Read the model definition and answer for the solid it produces. Units are mm, in the model's axes. A direction names the side the tool comes from. Coordinates: 2 decimals unless noted, no trailing zeros. Loops run counter-clockwise (first coordinate to the right, second up) from the corner with the lowest first, then second, coordinate; pieces in that order, holes last. Notation, with made-up numbers: (-28.5, 27) -> (18.5, 27) arc R29 cw to (18.5, 59) -> close; hole circle Ø10 at (16, -32). An arc over 180 degrees is marked (long way). Answer in a Markdown table with one row per item.
```python
from build123d import *
from build123d.topology import SkipClean

# Parameters (mm, degrees)
BOSS_EXTRUDE1_START   = 100
SKETCH2_R             = 5
BOSS_EXTRUDE1_DEPTH   = 130
SKETCH2_R_2           = 50
SKETCH2_R_3           = 45
BOSS_EXTRUDE1_2_DEPTH = 130
SKETCH3_R             = 100
SKETCH3_R_2           = 50
CUT_EXTRUDE1_DEPTH    = 60
BOSS_EXTRUDE3_START   = 60
SKETCH4_R             = 5
BOSS_EXTRUDE3_DEPTH   = 60


with BuildPart() as part:
    # Sketch2 → Boss-Extrude1 (new body)
    with BuildSketch(Plane(origin=(0, 0, 0), x_dir=(0, 0, -1), z_dir=(0.5372996083468277, 0.8433914458128833, 0)).offset(BOSS_EXTRUDE1_START)):
        with BuildLine():
            ThreePointArc((198.707774346, 59.213708116), (179.337427943, 57.550334456), (177.879118885, 38.163471214))
            ThreePointArc((177.879118885, 38.163471214), (179.755724079, 33.196743881), (178.825393945, 27.96945842))
            ThreePointArc((178.825393945, 27.96945842), (172.5, 0), (178.825393945, -27.96945842))
            ThreePointArc((178.825393945, -27.96945842), (179.755724079, -33.196743881), (177.879118885, -38.163471214))
            ThreePointArc((177.879118885, -38.163471214), (179.337427943, -57.550334456), (198.707774346, -59.213708116))
            ThreePointArc((198.707774346, -59.213708116), (203.694081302, -57.389764479), (208.911229611, -58.375356167))
            ThreePointArc((208.911229611, -58.375356167), (237.5, -65), (266.088770389, -58.375356167))
            ThreePointArc((266.088770389, -58.375356167), (271.305918698, -57.389764479), (276.292225654, -59.213708116))
            ThreePointArc((276.292225654, -59.213708116), (295.662572057, -57.550334456), (297.120881115, -38.163471214))
            ThreePointArc((297.120881115, -38.163471214), (295.244275921, -33.196743881), (296.174606055, -27.96945842))
            ThreePointArc((296.174606055, -27.96945842), (302.5, 0), (296.174606055, 27.96945842))
            ThreePointArc((296.174606055, 27.96945842), (295.244275921, 33.196743881), (297.120881115, 38.163471214))
            ThreePointArc((297.120881115, 38.163471214), (295.662572057, 57.550334456), (276.292225654, 59.213708116))
            ThreePointArc((276.292225654, 59.213708116), (271.305918698, 57.389764479), (266.088770389, 58.375356167))
            ThreePointArc((266.088770389, 58.375356167), (237.5, 65), (208.911229611, 58.375356167))
            ThreePointArc((208.911229611, 58.375356167), (203.694081302, 57.389764479), (198.707774346, 59.213708116))
        make_face()
        with Locations(Location((190, -47, 0), (0, 0, 90))):
            Circle(SKETCH2_R, mode=Mode.SUBTRACT)
        with Locations(Location((285, -47, 0), (0, 0, 90))):
            Circle(SKETCH2_R, mode=Mode.SUBTRACT)
        with Locations(Location((190, 47, 0), (0, 0, 90))):
            Circle(SKETCH2_R, mode=Mode.SUBTRACT)
        with Locations(Location((285, 47, 0), (0, 0, 90))):
            Circle(SKETCH2_R, mode=Mode.SUBTRACT)
        with BuildLine():
            ThreePointArc((195.584219919, 33.078200982), (192.883806526, 31.461344995), (190.819707243, 29.085224223))
            ThreePointArc((190.819707243, 29.085224223), (182.5, 0), (190.819707243, -29.085224223))
            ThreePointArc((190.819707243, -29.085224223), (192.883806526, -31.461344995), (195.584219919, -33.078200982))
            ThreePointArc((195.584219919, -33.078200982), (200.662572057, -36.449665544), (203.980110186, -41.56340923))
            ThreePointArc((203.980110186, -41.56340923), (205.568300645, -44.280780541), (207.922446674, -46.369907691))
            ThreePointArc((207.922446674, -46.369907691), (237.5, -55), (267.077553326, -46.369907691))
            ThreePointArc((267.077553326, -46.369907691), (269.431699355, -44.280780541), (271.019889814, -41.56340923))
            ThreePointArc((271.019889814, -41.56340923), (274.337427943, -36.449665544), (279.415780081, -33.078200982))
            ThreePointArc((279.415780081, -33.078200982), (282.116193474, -31.461344995), (284.180292757, -29.085224223))
            ThreePointArc((284.180292757, -29.085224223), (292.5, 0), (284.180292757, 29.085224223))
            ThreePointArc((284.180292757, 29.085224223), (282.116193474, 31.461344995), (279.415780081, 33.078200982))
            ThreePointArc((279.415780081, 33.078200982), (274.337427943, 36.449665544), (271.019889814, 41.56340923))
            ThreePointArc((271.019889814, 41.56340923), (269.431699355, 44.280780541), (267.077553326, 46.369907691))
            ThreePointArc((267.077553326, 46.369907691), (237.5, 55), (207.922446674, 46.369907691))
            ThreePointArc((207.922446674, 46.369907691), (205.568300645, 44.280780541), (203.980110186, 41.56340923))
            ThreePointArc((203.980110186, 41.56340923), (200.662572057, 36.449665544), (195.584219919, 33.078200982))
        make_face(mode=Mode.SUBTRACT)
    extrude(amount=BOSS_EXTRUDE1_DEPTH)

    # Sketch3 → Cut-Extrude1 (cut)
    with BuildSketch(Plane(origin=(53.729960835, 84.339144581, 0), x_dir=(0.8433914458128833, -0.5372996083468277, 0), z_dir=(-0.5372996083468277, -0.8433914458128833, 0))):
        with Locations((0, -237.5)):
            Circle(SKETCH3_R)
        with Locations(Location((0, -237.5, 0), (0, 0, 180))):
            Circle(SKETCH3_R_2, mode=Mode.SUBTRACT)
    extrude(amount=-CUT_EXTRUDE1_DEPTH, mode=Mode.SUBTRACT)



with BuildPart() as body_2:
    # Sketch2 → Boss-Extrude1 2 (new body)
    with BuildSketch(Plane(origin=(0, 0, 0), x_dir=(0, 0, -1), z_dir=(0.5372996083468277, 0.8433914458128833, 0)).offset(BOSS_EXTRUDE1_START)):
        with Locations(Location((237.5, 0, 0), (0, 0, 90))):
            Circle(SKETCH2_R_2)
        with Locations(Location((237.5, 0, 0), (0, 0, 90))):
            Circle(SKETCH2_R_3, mode=Mode.SUBTRACT)
    extrude(amount=BOSS_EXTRUDE1_2_DEPTH)


with BuildPart() as part_1:
    with SkipClean():  # the faces are left unmerged after this step: merging them gives an invalid solid
        add(part.part)

        add(body_2.part)  # Boss-Extrude3 merges body 2
        # Sketch4 → Boss-Extrude3 (add)
        # profile 1 of 4: a face of its own
        with BuildSketch(Plane(origin=(85.967937335, 134.94263133, 0), x_dir=(0.8433914458128833, -0.5372996083468277, 0), z_dir=(-0.5372996083468277, -0.8433914458128833, 0)).offset(BOSS_EXTRUDE3_START)):
            with BuildLine():
                ThreePointArc((-33.164183333, -184.206022338), (-57.550334456, -179.337427943), (-52.940059929, -203.773731813))
                ThreePointArc((-52.940059929, -203.773731813), (-46.613065404, -210.182422478), (-46.525893445, -219.187675212))
                ThreePointArc((-46.525893445, -219.187675212), (-35.16778152, -201.958093144), (-17.818975805, -190.782935652))
                ThreePointArc((-17.818975805, -190.782935652), (-26.822801925, -190.600477562), (-33.164183333, -184.206022338))
            make_face()
            with Locations(Location((-47, -190, 0), (0, 0, 180))):
                Circle(SKETCH4_R, mode=Mode.SUBTRACT)
        # profile 2 of 4: a face of its own
        with BuildSketch(Plane(origin=(85.967937335, 134.94263133, 0), x_dir=(0.8433914458128833, -0.5372996083468277, 0), z_dir=(-0.5372996083468277, -0.8433914458128833, 0)).offset(BOSS_EXTRUDE3_START)):
            with BuildLine():
                ThreePointArc((17.818975805, -190.782935652), (26.822801925, -190.600477562), (33.164183333, -184.206022338))
                ThreePointArc((33.164183333, -184.206022338), (57.550334456, -179.337427943), (52.940059929, -203.773731813))
                ThreePointArc((52.940059929, -203.773731813), (46.613065404, -210.182422478), (46.525893445, -219.187675212))
                ThreePointArc((46.525893445, -219.187675212), (35.16778152, -201.958093144), (17.818975805, -190.782935652))
            make_face()
            with Locations(Location((47, -190, 0), (0, 0, 180))):
                Circle(SKETCH4_R, mode=Mode.SUBTRACT)
        # profile 3 of 4: a face of its own
        with BuildSketch(Plane(origin=(85.967937335, 134.94263133, 0), x_dir=(0.8433914458128833, -0.5372996083468277, 0), z_dir=(-0.5372996083468277, -0.8433914458128833, 0)).offset(BOSS_EXTRUDE3_START)):
            with BuildLine():
                ThreePointArc((17.818975805, -284.217064348), (35.16778152, -273.041906856), (46.525893445, -255.812324788))
                ThreePointArc((46.525893445, -255.812324788), (46.613065404, -264.817577522), (52.940059929, -271.226268187))
                ThreePointArc((52.940059929, -271.226268187), (57.550334456, -295.662572057), (33.164183333, -290.793977662))
                ThreePointArc((33.164183333, -290.793977662), (26.822801925, -284.399522438), (17.818975805, -284.217064348))
            make_face()
            with Locations(Location((47, -285, 0), (0, 0, 180))):
                Circle(SKETCH4_R, mode=Mode.SUBTRACT)
        # profile 4 of 4: a face of its own
        with BuildSketch(Plane(origin=(85.967937335, 134.94263133, 0), x_dir=(0.8433914458128833, -0.5372996083468277, 0), z_dir=(-0.5372996083468277, -0.8433914458128833, 0)).offset(BOSS_EXTRUDE3_START)):
            with BuildLine():
                ThreePointArc((-17.818975805, -284.217064348), (-26.822801925, -284.399522438), (-33.164183333, -290.793977662))
                ThreePointArc((-33.164183333, -290.793977662), (-57.550334456, -295.662572057), (-52.940059929, -271.226268187))
                ThreePointArc((-52.940059929, -271.226268187), (-46.613065404, -264.817577522), (-46.525893445, -255.812324788))
                ThreePointArc((-46.525893445, -255.812324788), (-35.16778152, -273.041906856), (-17.818975805, -284.217064348))
            make_face()
            with Locations(Location((-47, -285, 0), (0, 0, 180))):
                Circle(SKETCH4_R, mode=Mode.SUBTRACT)
        extrude(amount=-BOSS_EXTRUDE3_DEPTH)


solid = part_1.part
```
1. Given pin 1 Ø3 at (y, z) = (133.5, -258.5) entering from +X; pin 2 Ø6 at (x, y) = (147.5, 135.5) entering from +Z; pin 3 Ø2 at (y, z) = (182.5, -271) entering from -X, each flat-ended and moving along its own axis, determine where each tip first touches the part or whether it passes through.
A:
| item | result |
|---|---|
| pin 1 | stops at x = 159.11 |
| pin 2 | stops at z = -175.09 |
| pin 3 | stops at x = 47.6 |
2. A cutting plane is placed at B-B on y = 140.5. Count the separate pieces of the cut face and the enclosed holes in it, and give its area (3 significant figures).
A:
| item | result |
|---|---|
| separate pieces | 2 |
| enclosed holes | 5 |
| area | 7,040 mm2 |
3. Find the intervals of material crossed by probe 1 along Z at (x, y) = (132, 133); probe 2 along X at (y, z) = (133, -247); probe 3 along X at (y, z) = (119, -269), in increasing order.
A:
| item | result |
|---|---|
| probe 1 | z = -298.2 to -271.8, -267.68 to -258.37, -216.63 to -207.32, -203.2 to -176.8 |
| probe 2 | x = 26.53 to 32.58, 136.88 to 142.93, 148.96 to 160.97 |
| probe 3 | x = 17.09 to 37.71, 113.92 to 121.85, 128.9 to 143.95 |
4. The mould has two halves that part along Y. Classify faces 1 (the flat face through (171.541, 163.425, -236.59)), 2 (the cylindrical face through (49.075, 163.295, -194.957)), 3 (the flat face through (134.82, 103.82, -236.96)): pulls with the +Y half, pulls with the -Y half, needs draft (parallel to the pull), parting line crosses it, or undercut.
A:
| item | result |
|---|---|
| face 1 | pulls with the +Y half |
| face 2 | undercut |
| face 3 | pulls with the -Y half |
5. A tool of negligible diameter and unlimited length cuts with its end or side. For faces 4 (the flat face through (116.153, 115.712, -273.528)), 5 (the flat face through (85.52, 135.23, -295.54)), 6 (the flat face through (36.9, 166.2, -237)), 7 (the flat face through (85.52, 135.23, -179.22)), from which of +Z, -Z, +X, -X, +Y, -Y can it reach the whole face along a straight path? Write none if from no direction.
A:
| item | result |
|---|---|
| face 4 | none |
| face 5 | -Z |
| face 6 | -X |
| face 7 | +Z |
6. A cutting plane is placed at A-A on z = -211.5. Give the vertices of the cut face in (x, y).
A:
| item | result |
|---|---|
| outline | (14.81, 109.14) -> (22.75, 104.07) -> (92.6, 213.71) -> (87.56, 216.93) -> (49.95, 157.89) -> (47.04, 159.74) -> close; (35.72, 166.95) -> (45.09, 160.98) -> (82.7, 220.02) -> (73.34, 225.99) -> close; (84.71, 64.6) -> (92.65, 59.54) -> (124.89, 110.14) -> (121.99, 112) -> (159.6, 171.03) -> (154.56, 174.25) -> close; (126.84, 108.9) -> (136.21, 102.93) -> (173.82, 161.97) -> (164.46, 167.94) -> close |
7. A cutting plane is placed at C-C on z = -251. Give the vertices of the cut face in (x, y), and give its area (3 significant figures).
A:
| item | result |
|---|---|
| outline | (13.13, 110.21) -> (17.53, 107.4) -> (87.37, 217.04) -> (82.98, 219.85) -> close; (32.34, 169.11) -> (41, 163.59) -> (78.61, 222.63) -> (69.95, 228.14) -> close; (89.93, 61.27) -> (94.33, 58.47) -> (164.18, 168.11) -> (159.78, 170.92) -> close; (130.94, 106.3) -> (139.59, 100.78) -> (177.2, 159.82) -> (168.55, 165.33) -> close |
| area | 2,790 mm2 |
